from build123d import *

# Parameters (mm, degrees)
F0_R     = 1.65
F0_R_2   = 1
F1_DEPTH = 4


with BuildPart() as f1:
    # F0 (on Top) → F1 (new body)
    with BuildSketch(Plane.XY):
        with BuildLine():
            ThreePointArc((-22.118284, 17.320522), (-13.456044, 23.902693), (-10.168284, 34.273324))
            ThreePointArc((-10.168284, 34.273324), (-38.538916, 48.985564), (-34.218284, 17.320522))
            Line((-34.218284, 17.320522), (-34.218284, 34.273324))
            ThreePointArc((-34.218284, 34.273324), (-28.168284, 40.323324), (-22.118284, 34.273324))
            Line((-22.118284, 34.273324), (-22.118284, 17.320522))
        make_face()
        with Locations((-38.993284, 28.023324)):
            Circle(F0_R, mode=Mode.SUBTRACT)
        with Locations((-17.343284, 28.023324)):
            Circle(F0_R, mode=Mode.SUBTRACT)
        with Locations((-38.993284, 40.523324)):
            Circle(F0_R, mode=Mode.SUBTRACT)
        with Locations((-28.168284, 46.773324)):
            Circle(F0_R_2, mode=Mode.SUBTRACT)
        with Locations((-17.343284, 40.523324)):
            Circle(F0_R, mode=Mode.SUBTRACT)
    extrude(amount=F1_DEPTH)


solid = f1.part
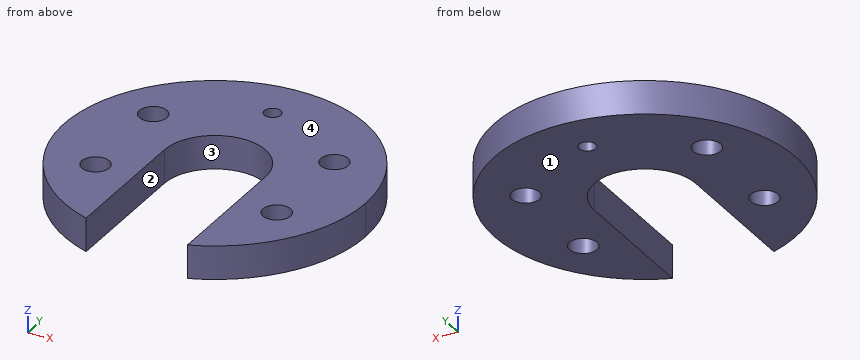
CAD build for the part. Positions are in the model's coordinates, mm. Face numbers are marked on the shaded views. A direction names the side the tool comes from. Round coordinates to 2 decimals unless told otherwise and drop trailing zeros. Order: outer loops, then holes, each group sorted by start corner. A loop starts at its lowest first (then second) coordinate and runs counter-clockwise, first axis right, second up. Notation, with made-up numbers: (47, 41) -> (94, 41) arc R4 ccw to (94, 47) -> close; hole circle Ø4 at (62.5, -8). An arc over 180 degrees is marked (long way). Write item = value, one per line. Start each with the question number.
(1) Pull direction X, two halves, no side cores. Call the marked faces 3 and 4: released by +X, released by -X, zero draft, split by the parting line, or undercut.
(2) Probe line 1 (Y direction, x = -38, z = 3.1); line 2 (Y direction, x = -16, z = 1.15); line 3 (Y direction, x = -29, z = 3.2). List the from-to ranges inside material, lowest first. Write a range as [from, to].
(3) Pin check, flat tips, straight feed: P1, Ø2.5, axis at x = -38.99, y = 28.02, coming from the -Z side; P2, Ø2, axis at y = 27.5, z = 2, coming from the -X side; P3, Ø2, axis at x = -26.5, z = 1.5, coming from the -Y side; P4, Ø1.5, axis at y = 30, z = 1.5, coming from the +X side. Stop position of each tip, or through.
(4) Cut at D-D, the plane y = 33.5. List the corners of the cut face in (x, z).
(5) Cut at B-B, the plane x = -38.5. List the corners of the cut face in (y, z).
(6) Which spindle directions (+Z, -Z, +X, -X, +Y, -Y) get a long thin tool onto all of the face, cutting with end or side? Do the marked faces 1 and 2. Say none if no direction does.
(7) Cut at A-A, the plane y = 38. List the corners of the cut face in (x, z).
(8) Cut at C-C, the plane z = 2.85. List the corners of the cut face in (x, y), then the cut area to 3 significant figures.
Model answer:
q1.face_3 = undercut
q1.face_4 = zero draft
q2.line_1 = [19.2, 26.71], [29.34, 39.21], [41.84, 49.35]
q2.line_2 = [21.01, 27.07], [28.98, 39.57], [41.48, 47.54]
q2.line_3 = [40.27, 46.22], [47.33, 52.25]
q3.P1 = through
q3.P2 = -45.22
q3.P3 = 39.7
q3.P4 = -10.52
q4.outline = (-46.15, 0) -> (-34.22, 0) -> (-34.22, 4) -> (-46.15, 4) -> close; (-22.12, 0) -> (-10.18, 0) -> (-10.18, 4) -> (-22.12, 4) -> close
q5.outline = (19.53, 0) -> (26.45, 0) -> (26.45, 4) -> (19.53, 4) -> close; (29.6, 0) -> (38.95, 0) -> (38.95, 4) -> (29.6, 4) -> close; (42.1, 0) -> (49.01, 0) -> (49.01, 4) -> (42.1, 4) -> close
q6.face_1 = -Z, +X, -X, +Y, -Y
q6.face_2 = +Z, -Z, -Y
q7.outline = (-45.78, 0) -> (-32.93, 0) -> (-32.93, 4) -> (-45.78, 4) -> close; (-23.4, 0) -> (-10.56, 0) -> (-10.56, 4) -> (-23.4, 4) -> close
q8.outline = (-34.22, 17.32) -> (-34.22, 34.27) arc R6.05 cw to (-22.12, 34.27) -> (-22.12, 17.32) arc R18 ccw (long way) to start; hole circle Ø3.3 at (-38.99, 28.02); hole circle Ø3.3 at (-38.99, 40.52); hole circle Ø2 at (-28.17, 46.77); hole circle Ø3.3 at (-17.34, 28.02); hole circle Ø3.3 at (-17.34, 40.52)
q8.area = 709 mm2
